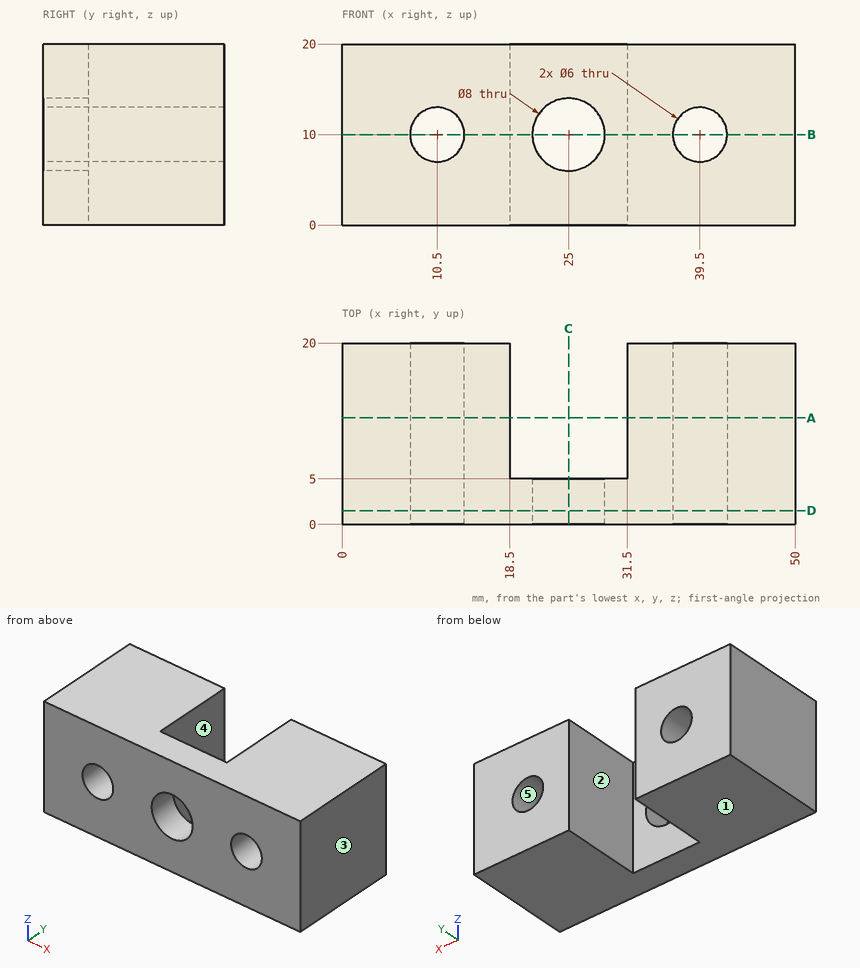
Check sheet for the drawn part. Datum: minimum x, y, z corner. Units: mm. A direction names the side the tool comes from. Give positions to 0.01 mm unless a question says otherwise; leave off trailing zeros. Order: outer loops, then holes, each group sorted by start corner. A loop starts at its lowest first (then second) coordinate and runs counter-clockwise, first axis right, second up. Notation, with made-up numbers: (5, 10) - (15, 10) arc R29 ccw to (15, 44) - close; hole circle Ø6 at (63.5, -11.75). An arc over 180 degrees is marked (long way). Answer as a JSON object with one key per item and string values.
(1) Tool access check on the marked faces 4 and 5. Record the directions out of +Z, -Z, +X, -X, +Y, -Y that give a thin tool (end or side, any length) a straight path to the whole face; none if there is none.
Report:
{"face 4": "+Z, -Z, +Y", "face 5": "+Y, -Y"}
(2) Cross-section at C-C (x = 25). Record the cut outline in (y, z), then the cut area to 3 significant figures.
Report:
{"outline": "(0, 0) - (5, 0) - (5, 6) - (0, 6) - close; (0, 14) - (5, 14) - (5, 20) - (0, 20) - close", "area": "60.0 mm^2"}
(3) Depth check by flat-ended pin: pin 1 Ø4 at (x, y) = (36.5, 10.5) entering from -Z; pin 2 Ø2 at (x, y) = (29.5, 15) entering from -Z; pin 3 Ø6.5 at (x, z) = (24, 12) entering from +Y. Enter the tip coordinate at first touch or a pass-through.
Report:
{"pin 1": "z = 0", "pin 2": "through", "pin 3": "y = 5"}
(4) Cross-section at D-D (y = 1.5). Record the cut outline in (x, z), then the cut area to 3 significant figures.
Report:
{"outline": "(0, 0) - (50, 0) - (50, 20) - (0, 20) - close; hole circle Ø6 at (10.5, 10); hole circle Ø8 at (25, 10); hole circle Ø6 at (39.5, 10)", "area": "893 mm^2"}
(5) Cross-section at B-B (z = 10). Record the cut outline in (x, y), then the cut area to 3 significant figures.
Report:
{"outline": "(0, 0) - (7.5, 0) - (7.5, 20) - (0, 20) - close; (13.5, 0) - (21, 0) - (21, 5) - (18.5, 5) - (18.5, 20) - (13.5, 20) - close; (29, 0) - (36.5, 0) - (36.5, 20) - (31.5, 20) - (31.5, 5) - (29, 5) - close; (42.5, 0) - (50, 0) - (50, 20) - (42.5, 20) - close", "area": "525 mm^2"}
(6) Draft check along X on the marked faces 1, 2 and 3. Enter one of: released by +X, released by -X, zero draft, split by the parting line, or undercut.
Report:
{"face 1": "zero draft", "face 2": "undercut", "face 3": "released by +X"}
(7) Material ranges on line 1 (X direction, y = 16.5, z = 10.25); line 2 (Z direction, x = 39.5, y = 5.5); line 3 (X direction, y = 11.75, z = 8.5), recorded low to high.
Report:
{"line 1": "0 to 7.51, 13.49 to 18.5, 31.5 to 36.51, 42.49 to 50", "line 2": "0 to 7, 13 to 20", "line 3": "0 to 7.9, 13.1 to 18.5, 31.5 to 36.9, 42.1 to 50"}
(8) Cross-section at A-A (y = 11.75). Record the cut outline in (x, z).
Report:
{"outline": "(0, 0) - (18.5, 0) - (18.5, 20) - (0, 20) - close; (31.5, 0) - (50, 0) - (50, 20) - (31.5, 20) - close; hole circle Ø6 at (10.5, 10); hole circle Ø6 at (39.5, 10)"}
